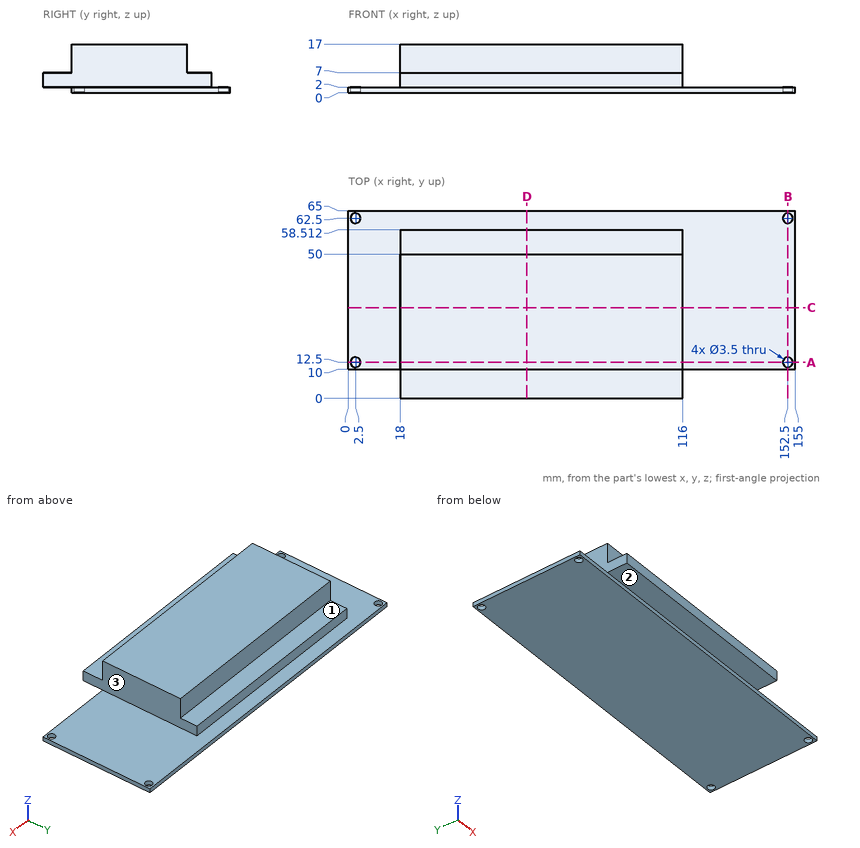
Drawing for the job (mm, zero at the part's lowest x, y, z). A direction names the side the tool comes from. Give positions to 0.01 mm unless a question says otherwise; leave off trailing zeros. Loops run counter-clockwise (first coordinate to the right, second up) from the corner with the lowest first, then second, coordinate; pieces in that order, holes last.
(1) Band-saw the part on B-B (x = 152.5). Write the cut outline in (y, z), and give its area (3 significant figures).
Return value:
outline: (10, 0) - (10.75, 0) - (10.75, 2) - (10, 2) - close; (14.25, 0) - (60.75, 0) - (60.75, 2) - (14.25, 2) - close; (64.25, 0) - (65, 0) - (65, 2) - (64.25, 2) - close
area: 96.0 mm2
(2) Band-saw the part on A-A (y = 12.5). Write the cut outline in (x, z), and give its area (3 significant figures).
Return value:
outline: (0, 0) - (0.75, 0) - (0.75, 2) - (0, 2) - close; (4.25, 0) - (150.75, 0) - (150.75, 2) - (116, 2) - (116, 17) - (18, 17) - (18, 2) - (4.25, 2) - close; (154.25, 0) - (155, 0) - (155, 2) - (154.25, 2) - close
area: 1,770 mm2
(3) 3-axis set-ups, long thin cutter, end or side, ignore diameter. For the marked faces 1, 2 and 3: which of +Z, -Z, +X, -X, +Y, -Y reach the whole face in a straight line?
Return value:
face 1: +Z, +X, -X, +Y
face 2: -Z, +X, -X, -Y
face 3: +Z, +X, +Y, -Y
(4) Drill centre lines: line 1 along Y through (x, z) = (152.5, 0.5); line 2 along Z through (x, y) = (99.5, 53); line 3 along X through (y, z) = (33, 8). Where is each one in solid material? Low to high.
Return value:
line 1: y = 10 to 10.75, 14.25 to 60.75, 64.25 to 65
line 2: z = 0 to 7
line 3: x = 18 to 116
(5) Pin check, flat tips, straight feed: pin 1 (3 mm diameter, centred on x = 152.5, y = 12.5, fed in from -Z); pin 2 (8 mm diameter, centred on x = 63, z = 2.5, fed in from +Y); pin 3 (2.5 mm diameter, centred on x = 86.5, z = 5, fed in from +Y); pin 4 (4.5 mm diameter, centred on y = 18, z = 7, fed in from -X). Stop position of each tip, or through.
Return value:
pin 1: passes through
pin 2: stops at y = 65
pin 3: stops at y = 58.51
pin 4: stops at x = 18
(6) Band-saw the part on C-C (y = 31.5). Write the cut outline in (x, z), and give its area (3 significant figures).
Return value:
outline: (0, 0) - (155, 0) - (155, 2) - (116, 2) - (116, 17) - (18, 17) - (18, 2) - (0, 2) - close
area: 1,780 mm2
(7) Band-saw the part on D-D (x = 62). Write the cut outline in (y, z), and give its area (3 significant figures).
Return value:
outline: (0, 2) - (10, 2) - (10, 0) - (65, 0) - (65, 2) - (58.51, 2) - (58.51, 7) - (50, 7) - (50, 17) - (10, 17) - (10, 7) - (0, 7) - close
area: 803 mm2
